Autodesk Inventor part; units mm, degrees
ref_plane "YZ Plane" through (0, 0, 0) normal (1, 0, 0) x (0, 1, 0)
ref_plane "XZ Plane" through (0, 0, 0) normal (0, 1, 0) x (-1, 0, 0)
ref_plane "XY Plane" through (0, 0, 0) normal (0, 0, 1) x (1, 0, 0)
sketch "Эскиз1" plane through (0, 0, 0) normal (0, 1, 0) x (-1, 0, 0)
  circle A0 centre (0, 0) radius 12.7
  circle A1 centre (0, 0) radius 15
  dimension "d0" = 25.4
  dimension "d1" = 30
extrude "Выдавливание1" add sketch "Эскиз1" along normal blind 17.5
sketch "Эскиз3" plane through (0, 17.5, 0) normal (0, 1, 0) x (1, 0, 0)
  circle A0 centre (0, 0) radius 15
  circle A1 centre (0, 0) radius 8.25
  circle A2 centre (0, 0) radius 15
  dimension "d4" = 16.5
  dimension "d9" = 0
extrude "Выдавливание2" add sketch "Эскиз3" along normal blind 30
fillet "Сопряжение1" radius 5 1 edges at (-8.25, 17.5, 0)
fillet "Сопряжение2" radius 1 2 edges at (0, 17.5, -12.7) (0, 17.5, 12.7)
Source: CAD feature listing. Evaluate the final solid. Frame: model axes, mm. A direction names the side the tool comes from. Give positions to 0.01 mm unless a question says otherwise; leave off trailing zeros. Loops run counter-clockwise (first coordinate to the right, second up) from the corner with the lowest first, then second, coordinate; pieces in that order, holes last. Notation, with made-up numbers: (-12.75, 57.5) -> (36.25, 57.5) arc R29 cw to (36.25, 86.5) -> close; hole circle Ø7 at (71.5, 32.25). An arc over 180 degrees is marked (long way). Use a Markdown table: item, result. Add a question column.
(1) Section query A-A (y = 33). Output: boundary loops of the cut face in (x, z), then the cut area to 3 significant figures.
(2) Access query for faces 4 (the face through (2.75, 8.22, 12.4)), 5 (the face through (11, 0, 7)). Directions: +Z, -Z, +X, -X, +Y, -Y. A direction counts if a zero-diameter tool reaches every point of the face in a straight line with its end or side. Return the directions, or none.
(3) First-contact query: pin 1 Ø1.5 at (x, y) = (-1, 41.5) entering from -Z; pin 2 Ø3 at (x, y) = (2.5, 12) entering from +Z; pin 3 Ø5 at (y, z) = (19, 3.5) entering from +X. Flat tips, straight axial feed; report the tip coordinate or a pass-through.
(4) Pull-direction query (X, two-part tool) for faces 1 (the face through (7.62, 34.81, -3.16)), 2 (the face through (0.989, 23.418, 14.967)), 3 (the face through (6, 47.5, 6)); classes: +X half, -X half, draft (parallel to the pull), parting line (faces both ways), or undercut.
(5) Ray query, line 1 (Z direction, x = 0, y = 6.25); line 2 (X direction, y = 38.5, z = 0). Return the intervals inside material, ascending.
Checked values:
| question | item | result |
|---|---|---|
| 1 | outline | circle Ø30 at (0, 0); hole circle Ø16.5 at (0, 0) |
| 1 | area | 493 mm^2 |
| 2 | face 4 | -Y |
| 2 | face 5 | +Z, -Z, +X, -X, -Y |
| 3 | pin 1 | z = -15 |
| 3 | pin 2 | z = 14.97 |
| 3 | pin 3 | x = 14.97 |
| 4 | face 1 | undercut |
| 4 | face 2 | parting line |
| 4 | face 3 | draft |
| 5 | line 1 | -15 to -12.7, 12.7 to 15 |
| 5 | line 2 | -15 to -8.25, 8.25 to 15 |
